Verification items for the finished model (mm, model axes). Coordinates: 2 decimals unless noted, no trailing zeros. Order: outer loops, then holes, each group sorted by start corner. A loop starts at its lowest first (then second) coordinate and runs counter-clockwise, first axis right, second up. Notation, with made-up numbers: (-15.75, 51) -> (-1.75, 51) arc R23 cw to (-1.75, 64) -> close; hole circle Ø8 at (22, 13.5). An arc over 180 degrees is marked (long way). Write item = value, one per line. Start each with the question number.
1. Cross-section at C-C on z = 1.6. Record the cut outline in (x, y).
2. Thickness scan on line 1 along Y through (x, z) = (0, 0.4); line 2 along Y through (x, z) = (2, 0.9); line 3 along X through (y, z) = (-1.25, 1.7). Record the ranges inside material, lowest first. Write a range as from..to.
3. Cross-section at A-A on x = 0. Record the cut outline in (y, z), plus the area to 3 significant figures.
from build123d import *

# Parameters (mm, degrees)
SKETCH2_R           = 9
SKETCH2_R_2         = 3
BOSS_EXTRUDE1_DEPTH = 2
SKETCH4_R           = 9
BOSS_EXTRUDE2_DEPTH = 0.1
BOSS_EXTRUDE2_TAPER = 86.7
SKETCH5_R           = 3
CUT_EXTRUDE1_DEPTH  = 0.1


with BuildPart() as part:
    # Sketch2 → Boss-Extrude1 (new body)
    with BuildSketch(Plane.XY):
        Circle(SKETCH2_R)
        Circle(SKETCH2_R_2, mode=Mode.SUBTRACT)
    extrude(amount=BOSS_EXTRUDE1_DEPTH)

    # Sketch4 → Boss-Extrude2 (add)
    with BuildSketch(Plane.XY.offset(2)):
        Circle(SKETCH4_R)
    extrude(amount=BOSS_EXTRUDE2_DEPTH, taper=BOSS_EXTRUDE2_TAPER)

    # Sketch5 → Cut-Extrude1 (cut)
    with BuildSketch(Plane(origin=(0, 0, 2), x_dir=(-1, 0, 0), z_dir=(0, 0, -1))):
        Circle(SKETCH5_R)
    extrude(amount=-CUT_EXTRUDE1_DEPTH, mode=Mode.SUBTRACT)


solid = part.part
Worked out:
q1.outline = circle Ø18 at (0, 0); hole circle Ø6 at (0, 0)
q2.line_1 = -9..-3, 3..9
q2.line_2 = -8.77..-2.24, 2.24..8.77
q2.line_3 = -8.91..-2.73, 2.73..8.91
q3.outline = (-9, 0) -> (-3, 0) -> (-3, 2.1) -> (-7.27, 2.1) -> (-9, 2) -> close; (3, 0) -> (9, 0) -> (9, 2) -> (7.27, 2.1) -> (3, 2.1) -> close
q3.area = 25.0 mm²
